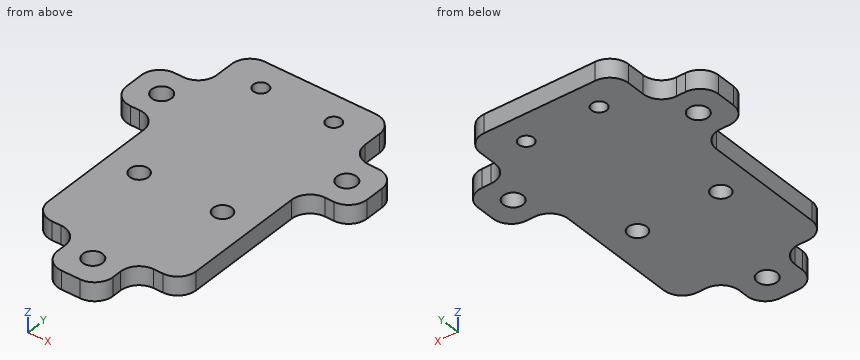
from build123d import *

# Parameters (mm, degrees)
SKETCH1_W                   = 50.8
SKETCH1_H                   = 101.6
BOSS_EXTRUDE1_DEPTH         = 6.35
F_7_0_201_DIAMETER_HOLE1_D  = 5.1054
SKETCH4_W                   = 15.875
SKETCH4_H                   = 19.05
SKETCH4_W_2                 = 19.05
SKETCH4_H_2                 = 15.875
BOSS_EXTRUDE2_DEPTH         = 6.35
F_1_4_CLEARANCE_HOLE1_D     = 6.7564
SKETCH7_W                   = 50.8
SKETCH7_H                   = 9.525
CUT_EXTRUDE1_DEPTH          = 122.689926144
FILLET1_R                   = 6.35
F_1_4_0_25_DIAMETER_HOLE1_D = 6.35


with BuildPart() as part:
    # Sketch1 → Boss-Extrude1 (new body)
    with BuildSketch(Plane.XY):
        with Locations((25.4, 50.8)):
            Rectangle(SKETCH1_W, SKETCH1_H)
    extrude(amount=BOSS_EXTRUDE1_DEPTH)

    # #7 (0.201) Diameter Hole1 (through all)
    with Locations(Plane.XY.offset(6.35)):
        with Locations((12.899999981, 82.13900006), (37.900000019, 82.13900006)):
            Hole(F_7_0_201_DIAMETER_HOLE1_D / 2)

    # Sketch4 → Boss-Extrude2 (add)
    with BuildSketch(Plane.XY.offset(6.35)):
        with Locations((-7.9375, 63.5)):
            Rectangle(SKETCH4_W, SKETCH4_H)
        with Locations((58.7375, 63.5)):
            Rectangle(SKETCH4_W, SKETCH4_H)
        with Locations((25.4, -7.9375)):
            Rectangle(SKETCH4_W_2, SKETCH4_H_2)
    extrude(amount=-BOSS_EXTRUDE2_DEPTH)

    # 1/4 Clearance Hole1 (through all)
    with Locations(Plane.XY.offset(6.35)):
        with Locations((-6.35, 63.5), (57.15, 63.5), (25.4, -6.35)):
            Hole(F_1_4_CLEARANCE_HOLE1_D / 2)

    # Sketch7 → Cut-Extrude1 (cut, through all)
    with BuildSketch(Plane(origin=(0, 0, 0), x_dir=(-1, 0, 0), z_dir=(0, 0, -1))):
        with Locations((-25.4, 96.8375)):
            Rectangle(SKETCH7_W, SKETCH7_H)
    extrude(amount=-CUT_EXTRUDE1_DEPTH, mode=Mode.SUBTRACT)

    # Fillet1
    fillet1_edges = [part.edges().sort_by_distance(p)[0] for p in [
        (-15.875, 73.025, 3.175),
        (-15.875, 53.975, 3.175),
        (0, 53.975, 3.175),
        (0, 73.025, 3.175),
        (50.8, 53.975, 3.175),
        (66.675, 53.975, 3.175),
        (66.675, 73.025, 3.175),
        (50.8, 73.025, 3.175),
        (34.925, -15.875, 3.175),
        (34.925, 0, 3.175),
        (15.875, 0, 3.175),
        (15.875, -15.875, 3.175),
        (50.8, 0, 3.175),
        (0, 0, 3.175),
        (50.8, 92.075, 3.175),
        (0, 92.075, 3.175),
    ]]
    fillet(fillet1_edges, radius=FILLET1_R)

    # 1/4 (0.25) Diameter Hole1 (through all)
    with Locations(Plane(origin=(0, 0, 0), x_dir=(-1, 0, 0), z_dir=(0, 0, -1))):
        with Locations((-39.6875, 31.75), (-11.1125, 31.75)):
            Hole(F_1_4_0_25_DIAMETER_HOLE1_D / 2)


solid = part.part
The listing builds one solid part. Answer for the finished solid, in the listing's coordinates (mm). Round coordinates to 2 decimals unless told otherwise and drop trailing zeros. Write each loop counter-clockwise with the first axis right and the second up, starting at its lowest first coordinate (ties: lowest second). Pieces come first, ordered by that corner, then holes. Notation, with made-up numbers: (49.25, -19.75) - (71.25, -19.75) arc R9 cw to (71.25, -9.75) - close; hole circle Ø8 at (42, 48.25). An arc over 180 degrees is marked (long way). Use one line per item in the form item = value. Start each with the question number.
Item 1: A cutting plane is placed at C-C (y = 63.5). Write down the section's boundary in (x, z) (3 decimals), plus the area to 3 significant figures.
Item 2: Find the intervals of material crossed by line 1 (Y direction, x = 57.15, z = 1.5) (3 decimals); line 2 (Y direction, x = 37.9, z = 4.75) (3 decimals); line 3 (Y direction, x = 29, z = 0.5) (3 decimals), in increasing order. Write a range as [from, to].
Item 3: A cutting plane is placed at D-D (x = 56). Write down the section's boundary in (y, z).
Item 4: A cutting plane is placed at B-B (x = 25.4). Write down the section's boundary in (y, z) (3 decimals), plus the area to 3 significant figures.
Item 5: A cutting plane is placed at A-A (y = 31.75). Write down the section's boundary in (x, z).
Item 6: Flat-ended cylindrical pins translate along their axes: pin 1 Ø1 at (x, z) = (2.5, 1) entering from +Y; pin 2 Ø1.9 at (y, z) = (81.5, 4.5) entering from +X; pin 3 Ø1.6 at (x, z) = (42.5, 4) entering from -Y; pin 4 Ø7.5 at (x, y) = (39.69, 31.75) entering from +Z. Find the tip coordinate at first contact, or state that the pin passes through.
The answers:
q1.outline = (-15.875, 0) - (-9.728, 0) - (-9.728, 6.35) - (-15.875, 6.35) - close; (-2.972, 0) - (53.772, 0) - (53.772, 6.35) - (-2.972, 6.35) - close; (60.528, 0) - (66.675, 0) - (66.675, 6.35) - (60.528, 6.35) - close
q1.area = 438 mm^2
q2.line_1 = [53.975, 60.122], [66.878, 73.025]
q2.line_2 = [-0.971, 29.126], [34.374, 79.586], [84.692, 92.075]
q2.line_3 = [-15.861, 92.075]
q3.outline = (53.87, 0) - (60.32, 0) - (60.32, 6.35) - (53.87, 6.35) - close; (66.68, 0) - (73.13, 0) - (73.13, 6.35) - (66.68, 6.35) - close
q4.outline = (-15.875, 0) - (-9.728, 0) - (-9.728, 6.35) - (-15.875, 6.35) - close; (-2.972, 0) - (92.075, 0) - (92.075, 6.35) - (-2.972, 6.35) - close
q4.area = 643 mm^2
q5.outline = (0, 0) - (7.94, 0) - (7.94, 6.35) - (0, 6.35) - close; (14.29, 0) - (36.51, 0) - (36.51, 6.35) - (14.29, 6.35) - close; (42.86, 0) - (50.8, 0) - (50.8, 6.35) - (42.86, 6.35) - close
q6.pin_1 = 91.12
q6.pin_2 = 50.8
q6.pin_3 = 0
q6.pin_4 = 6.35
